```python
from build123d import *

# Parameters (mm, degrees)
F0_W      = 1219.2
F0_H      = 609.6
F1_DEPTH  = 609.6
F2_W      = 1168.4
F2_H      = 1168.4
F3_DEPTH  = 584.2
F4_W      = 1168.4
F4_H      = 25.4
F5_DEPTH  = 38.1
F7_DEPTH  = 12.7
F9_DEPTH  = 12.7
F11_DEPTH = 12.7


with BuildPart() as f1:
    # F0 (on Front) → F1 (new body, symmetric)
    with BuildSketch(Plane.XZ):
        Rectangle(F0_W, F0_H)
    extrude(amount=F1_DEPTH, both=True)

    # F2 (on face) → F3 (cut)
    with BuildSketch(Plane.XY.offset(304.8)):
        Rectangle(F2_W, F2_H)
    extrude(amount=-F3_DEPTH, mode=Mode.SUBTRACT)

    # F4 (on face) → F5 (cut)
    with BuildSketch(Plane.XY.offset(304.8)):
        with Locations((0, -596.9)):
            Rectangle(F4_W, F4_H)
    extrude(amount=-F5_DEPTH, mode=Mode.SUBTRACT)

    # F6 (on face) → F7 (cut)
    with BuildSketch(Plane.YZ.offset(-584.2)):
        Polygon((-609.6, 292.1), (-609.6, 266.7), (-584.2, 266.7), (584.2, 266.7), (584.2, 292.1), align=None)
    extrude(amount=-F7_DEPTH, mode=Mode.SUBTRACT)

    # F8 (on face) → F9 (cut)
    with BuildSketch(Plane.XZ.offset(-584.2)):
        Polygon((-596.9, 292.1), (-596.9, 266.7), (-584.2, 266.7), (584.2, 266.7), (584.2, 292.1), (-584.2, 292.1), align=None)
    extrude(amount=-F9_DEPTH, mode=Mode.SUBTRACT)

    # F10 (on face) → F11 (cut)
    with BuildSketch(Plane(origin=(584.2, 0, 0), x_dir=(0, -1, 0), z_dir=(-1, 0, 0))):
        Polygon((-596.9, 292.1), (-596.9, 266.7), (-584.2, 266.7), (584.2, 266.7), (609.6, 266.7), (609.6, 292.1), (-584.2, 292.1), align=None)
    extrude(amount=-F11_DEPTH, mode=Mode.SUBTRACT)


solid = f1.part
```
Can you work these out from the model? Positions are in its coordinate system, mm. A direction names the side the tool comes from. Round coordinates to 2 decimals unless told otherwise and drop trailing zeros. Loops run counter-clockwise (first coordinate to the right, second up) from the corner with the lowest first, then second, coordinate; pieces in that order, holes last. Notation, with made-up numbers: M -2.75,48 L 50.25,48 A27 ccw 50.25,71 Z; hole C 10.25,36.5 d3. An arc over 180 degrees is marked long. Answer as a JSON object with one key per item and string values. Group by question number.
Q1. Please list where these lines run through material, in increasing order: L1, parallel to X at y = -507, z = 149; L2, parallel to Z at x = 142.5, y = 482.5.
Q2. Imagine slicing it at A-A, the plane z = -254.5. Please give me the cut outline in (x, y).
Q3. Will these pins go through, and if not, where does the flat tip stop? pin 1 (4 mm diameter, centred on x = 259.5, z = 298, fed in from -Y); pin 2 (1.5 mm diameter, centred on x = 109.5, y = -477.5, fed in from +Z).
Q4. On a 3-axis mill with a long thin cutter (end or side, diameter ignored), from which of +Z, -Z, +X, -X, +Y, -Y can I reach the whole of each face in a straight line? I mean faces 1 (the flat face through (-590, -3, 304.8)), 2 (the flat face through (-8, 8, -279.4)). Say none if no direction works.
Q5. Imagine slicing it at B-B, the plane x = 416.5. Please give me the cut outline in (y, z).
Q6. Imagine slicing it at C-C, the plane y = 438. Please give me the cut outline in (x, z).
Findings:
{
 "1": {"L1": "x = -609.6 to -584.2, 584.2 to 609.6", "L2": "z = -304.8 to -279.4"},
 "2": {"outline": "M -609.6,-609.6 L 609.6,-609.6 L 609.6,609.6 L -609.6,609.6 Z; hole M -584.2,-584.2 L 584.2,-584.2 L 584.2,584.2 L -584.2,584.2 Z"},
 "3": {"pin 1": "stops at y = 584.2", "pin 2": "stops at z = -279.4"},
 "4": {"face 1": "+Z, +X, -X, +Y, -Y", "face 2": "+Z"},
 "5": {"outline": "M -609.6,-304.8 L 609.6,-304.8 L 609.6,304.8 L 584.2,304.8 L 584.2,292.1 L 596.9,292.1 L 596.9,266.7 L 584.2,266.7 L 584.2,-279.4 L -584.2,-279.4 L -584.2,266.7 L -609.6,266.7 Z"},
 "6": {"outline": "M -609.6,-304.8 L 609.6,-304.8 L 609.6,304.8 L 584.2,304.8 L 584.2,292.1 L 596.9,292.1 L 596.9,266.7 L 584.2,266.7 L 584.2,-279.4 L -584.2,-279.4 L -584.2,266.7 L -596.9,266.7 L -596.9,292.1 L -584.2,292.1 L -584.2,304.8 L -609.6,304.8 Z"}
}
